Work out the finished part from the listing and answer in its coordinate system (mm). Face numbers are marked on the shaded views. A direction names the side the tool comes from. Coordinates: 2 decimals unless noted, no trailing zeros. Write each loop counter-clockwise with the first axis right and the second up, starting at its lowest first coordinate (ties: lowest second). Pieces come first, ordered by that corner, then holes. Notation, with made-up numbers: (47, 80.5) - (62, 80.5) arc R18 cw to (62, 109.5) - close; hole circle Ø6 at (51.5, -20.5). An arc over 180 degrees is marked (long way). Use one line per item in the form item = value. Start each with the question number.
Item 1: For the marked faces 1 and 2, determine the directions among +Z, -Z, +X, -X, +Y, -Y from which every point of the face is accessible in a straight line to the end or side of a thin tool.
Item 2: A cutting plane is placed at B-B (y = -5.08). Write down the section's boundary in (x, z) (3 decimals).
Item 3: A cutting plane is placed at A-A (z = 3.45). Write down the section's boundary in (x, y) (3 decimals), then the cut area to 3 significant figures.
Item 4: A cutting plane is placed at C-C (z = 1.6). Write down the section's boundary in (x, y) (3 decimals).
Item 5: Consider probe 1 along Y at (x, z) = (-11.25, 1.5); probe 2 along Z at (x, y) = (-0.75, -9.5); probe 3 along X at (y, z) = (-7, 2.95). Determine where each line is inside the solid, lowest interval first.
Item 6: Given pin 1 (1.3 mm diameter, centred on x = 10.795, y = 9.525, fed in from -Z), flat-ended and moving along its own axis, determine where the tip first touches the part or whether it passes through.
Item 7: A cutting plane is placed at D-D (x = 11.5). Write down the section's boundary in (y, z), then the cut area to 3 significant figures.
Item 8: Determine the mould class of the marked faces 3, 4 and 5 for opening direction Y: released by +Y, released by -Y, zero draft, split by the parting line, or undercut.
from build123d import *

# Parameters (mm, degrees)
SKETCH1_R           = 2.1
SKETCH1_R_2         = 1.1
BOSS_EXTRUDE1_DEPTH = 2.5
BOSS_EXTRUDE2_START = 2.5
SKETCH1_3_R         = 2.1
SKETCH1_3_R_2       = 1.1
BOSS_EXTRUDE2_DEPTH = 2


with BuildPart() as part:
    # Sketch1 → Boss-Extrude1 (new body)
    # profile 1 of 5: a face of its own
    with BuildSketch(Plane.XY):
        with BuildLine():
            Line((10.795, 13.065), (-10.795, 13.065))
            ThreePointArc((-10.795, 13.065), (-13.298158005, 12.028158005), (-14.335, 9.525))
            Line((-14.335, 9.525), (-14.335, -9.525))
            ThreePointArc((-14.335, -9.525), (-13.298158005, -12.028158005), (-10.795, -13.065))
            Line((-10.795, -13.065), (10.795, -13.065))
            ThreePointArc((10.795, -13.065), (13.298158005, -12.028158005), (14.335, -9.525))
            Line((14.335, -9.525), (14.335, 9.525))
            ThreePointArc((14.335, 9.525), (13.298158005, 12.028158005), (10.795, 13.065))
        make_face()
        with Locations((10.795, 9.525)):
            Circle(SKETCH1_R, mode=Mode.SUBTRACT)
        with Locations((10.795, -5.08)):
            Circle(SKETCH1_R, mode=Mode.SUBTRACT)
        with Locations((-10.795, -5.08)):
            Circle(SKETCH1_R, mode=Mode.SUBTRACT)
        with Locations((-10.795, 9.525)):
            Circle(SKETCH1_R, mode=Mode.SUBTRACT)
    # profile 2 of 5: a face of its own
    with BuildSketch(Plane.XY):
        with Locations((-10.795, -5.08)):
            Circle(SKETCH1_R)
        with Locations((-10.795, -5.08)):
            Circle(SKETCH1_R_2, mode=Mode.SUBTRACT)
    # profile 3 of 5: a face of its own
    with BuildSketch(Plane.XY):
        with Locations((-10.795, 9.525)):
            Circle(SKETCH1_R)
        with Locations((-10.795, 9.525)):
            Circle(SKETCH1_R_2, mode=Mode.SUBTRACT)
    # profile 4 of 5: a face of its own
    with BuildSketch(Plane.XY):
        with Locations((10.795, 9.525)):
            Circle(SKETCH1_R)
        with Locations((10.795, 9.525)):
            Circle(SKETCH1_R_2, mode=Mode.SUBTRACT)
    # profile 5 of 5: a face of its own
    with BuildSketch(Plane.XY):
        with Locations((10.795, -5.08)):
            Circle(SKETCH1_R)
        with Locations((10.795, -5.08)):
            Circle(SKETCH1_R_2, mode=Mode.SUBTRACT)
    extrude(amount=BOSS_EXTRUDE1_DEPTH)

    # Sketch1<3> → Boss-Extrude2 (add)
    # profile 1 of 4: a face of its own
    with BuildSketch(Plane.XY.offset(BOSS_EXTRUDE2_START)):
        with Locations((-10.795, 9.525)):
            Circle(SKETCH1_3_R)
        with Locations((-10.795, 9.525)):
            Circle(SKETCH1_3_R_2, mode=Mode.SUBTRACT)
    # profile 2 of 4: a face of its own
    with BuildSketch(Plane.XY.offset(BOSS_EXTRUDE2_START)):
        with Locations((10.795, 9.525)):
            Circle(SKETCH1_3_R)
        with Locations((10.795, 9.525)):
            Circle(SKETCH1_3_R_2, mode=Mode.SUBTRACT)
    # profile 3 of 4: a face of its own
    with BuildSketch(Plane.XY.offset(BOSS_EXTRUDE2_START)):
        with Locations((10.795, -5.08)):
            Circle(SKETCH1_3_R)
        with Locations((10.795, -5.08)):
            Circle(SKETCH1_3_R_2, mode=Mode.SUBTRACT)
    # profile 4 of 4: a face of its own
    with BuildSketch(Plane.XY.offset(BOSS_EXTRUDE2_START)):
        with Locations((-10.795, -5.08)):
            Circle(SKETCH1_3_R)
        with Locations((-10.795, -5.08)):
            Circle(SKETCH1_3_R_2, mode=Mode.SUBTRACT)
    extrude(amount=BOSS_EXTRUDE2_DEPTH)


solid = part.part
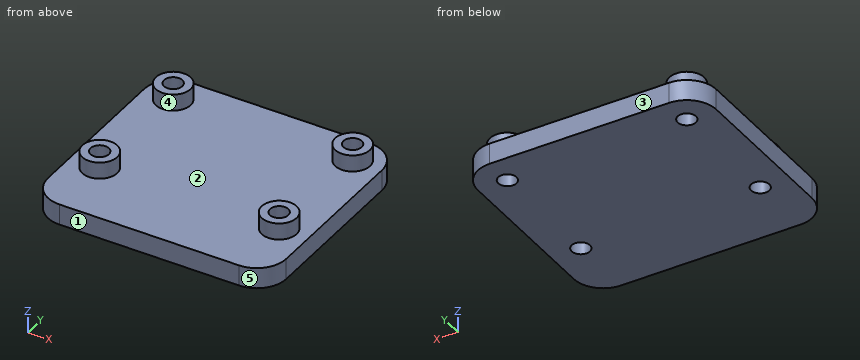
Answer:
q1.face_1 = +Z, -Z, +X, -X, -Y
q1.face_2 = +Z
q2.outline = (-14.335, 0) - (-11.895, 0) - (-11.895, 4.5) - (-12.895, 4.5) - (-12.895, 2.5) - (-14.335, 2.5) - close; (-9.695, 0) - (9.695, 0) - (9.695, 4.5) - (8.695, 4.5) - (8.695, 2.5) - (-8.695, 2.5) - (-8.695, 4.5) - (-9.695, 4.5) - close; (11.895, 0) - (14.335, 0) - (14.335, 2.5) - (12.895, 2.5) - (12.895, 4.5) - (11.895, 4.5) - close
q3.outline = circle Ø4.2 at (-10.795, -5.08); circle Ø4.2 at (-10.795, 9.525); circle Ø4.2 at (10.795, -5.08); circle Ø4.2 at (10.795, 9.525); hole circle Ø2.2 at (-10.795, -5.08); hole circle Ø2.2 at (-10.795, 9.525); hole circle Ø2.2 at (10.795, -5.08); hole circle Ø2.2 at (10.795, 9.525)
q3.area = 40.2 mm²
q4.outline = (-14.335, -9.525) arc R3.54 ccw to (-10.795, -13.065) - (10.795, -13.065) arc R3.54 ccw to (14.335, -9.525) - (14.335, 9.525) arc R3.54 ccw to (10.795, 13.065) - (-10.795, 13.065) arc R3.54 ccw to (-14.335, 9.525) - close; hole circle Ø2.2 at (-10.795, -5.08); hole circle Ø2.2 at (-10.795, 9.525); hole circle Ø2.2 at (10.795, -5.08); hole circle Ø2.2 at (10.795, 9.525)
q5.probe_1 = -13.04 to -6.08, -4.08 to 8.52, 10.53 to 13.04
q5.probe_2 = 0 to 2.5
q5.probe_3 = -11.65 to -9.94, 9.94 to 11.65
q6.pin_1 = through
q7.outline = (-12.99, 0) - (-5.92, 0) - (-5.92, 4.5) - (-7.06, 4.5) - (-7.06, 2.5) - (-12.99, 2.5) - close; (-4.24, 0) - (8.68, 0) - (8.68, 4.5) - (7.55, 4.5) - (7.55, 2.5) - (-3.1, 2.5) - (-3.1, 4.5) - (-4.24, 4.5) - close; (10.37, 0) - (12.99, 0) - (12.99, 2.5) - (11.5, 2.5) - (11.5, 4.5) - (10.37, 4.5) - close
q7.area = 65.6 mm²
q8.face_3 = released by +Y
q8.face_4 = undercut
q8.face_5 = released by -Y
